```python
from build123d import *

# Parameters (mm, degrees)
ANGLE_BRACKET_DEPTH = 24.765
CORNERS_R           = 5.08
SKETCH2_R           = 2.2225
HOLES_DEPTH         = 32.661678194
SLOTS_DEPTH         = 32.710646251


with BuildPart() as part:
    # Sketch1 → Angle Bracket (new body)
    with BuildSketch(Plane.XY):
        with BuildLine():
            Line((0, 13.589), (0, 1.27))
            ThreePointArc((0, 1.27), (0.371974388, 0.371974388), (1.27, 0))
            Line((1.27, 0), (15.24, 0))
            Line((15.24, 0), (15.24, 0.9398))
            Line((15.24, 0.9398), (1.8796, 0.9398))
            ThreePointArc((1.8796, 0.9398), (1.215061047, 1.215061047), (0.9398, 1.8796))
            Line((0.9398, 1.8796), (0.9398, 13.589))
            Line((0.9398, 13.589), (0, 13.589))
        make_face()
    extrude(amount=-ANGLE_BRACKET_DEPTH)

    # Corners
    corners_edges = [part.edges().sort_by_distance(p)[0] for p in [
        (0.4699, 13.589, 0),
        (15.24, 0.4699, -24.765),
        (0.4699, 13.589, -24.765),
        (15.24, 0.4699, 0),
    ]]
    fillet(corners_edges, radius=CORNERS_R)

    # Sketch2 → Holes (cut, through all)
    with BuildSketch(Plane(origin=(0.9398, 0, 0), x_dir=(0, 0, -1), z_dir=(1, 0, 0))):
        with Locations(Location((6.0325, 7.5565, 0), (0, 0, 90))):
            Circle(SKETCH2_R)
        with Locations(Location((18.7325, 7.5565, 0), (0, 0, 90))):
            Circle(SKETCH2_R)
    extrude(amount=-HOLES_DEPTH, mode=Mode.SUBTRACT)

    # Sketch3 → Slots (cut, through all)
    with BuildSketch(Plane(origin=(0, 0.9398, 0), x_dir=(-1, 0, 0), z_dir=(0, 1, 0))):
        with BuildLine():
            Line((-5.3975, -3.81), (-9.2075, -3.81))
            ThreePointArc((-9.2075, -3.81), (-11.43, -6.0325), (-9.2075, -8.255))
            Line((-9.2075, -8.255), (-5.3975, -8.255))
            ThreePointArc((-5.3975, -8.255), (-3.175, -6.0325), (-5.3975, -3.81))
        make_face()
        with BuildLine():
            Line((-5.3975, -16.51), (-9.2075, -16.51))
            ThreePointArc((-9.2075, -16.51), (-11.43, -18.7325), (-9.2075, -20.955))
            Line((-9.2075, -20.955), (-5.3975, -20.955))
            ThreePointArc((-5.3975, -20.955), (-3.175, -18.7325), (-5.3975, -16.51))
        make_face()
    extrude(amount=-SLOTS_DEPTH, mode=Mode.SUBTRACT)


solid = part.part
```
Source: CAD feature listing. Evaluate the final solid. Frame: model axes, mm. A direction names the side the tool comes from. Round coordinates to 2 decimals unless told otherwise and drop trailing zeros. Order: outer loops, then holes, each group sorted by start corner. A loop starts at its lowest first (then second) coordinate and runs counter-clockwise, first axis right, second up. Notation, with made-up numbers: (68, 17) -> (114, 17) arc R33 cw to (114, 52) -> close; hole circle Ø1 at (38, 34.5). An arc over 180 degrees is marked (long way). One line per item, written item: value. Start each with the question number.
Q1. Access query for faces 4 (the flat face through (2.8, 0.5, 0)), 5 (the flat face through (7.3, 0.5, -3.81)). Directions: +Z, -Z, +X, -X, +Y, -Y. A direction counts if a zero-diameter tool reaches every point of the face in a straight line with its end or side. Return the directions, or none.
Q2. Section query A-A (x = 6.5). Return the cut outline in (y, z) (3 decimals), plus the area to 3 significant figures.
Q3. Section query C-C (y = 9). Return the cut outline in (x, z).
Q4. Section query D-D (z = -11.5). Return the cut outline in (x, y).
Q5. Material intervals for probe 1 along X at (y, z) = (4.5, -19.75); probe 2 along Y at (x, z) = (1.5, -8.25), sorted ascending.
Q6. Pin query (flat end, axial travel): pin 1 (3 mm diameter, centred on y = 5, z = -10.5, fed in from +X); pin 2 (4 mm diameter, centred on y = 7.56, z = -6.03, fed in from +X); pin 3 (1 mm diameter, centred on x = 7.5, z = -8.5, fed in from +Y). Return the tip coordinate at first contact, or that it passes through.
Q7. Draft query along X for faces 1 (the flat face through (7.3, 0.5, -20.955)), 2 (the flat face through (0.94, 8, -12)), 3 (the flat face through (9, 0.94, -12)). Return one class per face: pulls with the +X half, pulls with the -X half, needs draft (parallel to the pull), parting line crosses it, or undercut.
Q8. Section query B-B (z = -17.5). Return the cut outline in (x, y), plus the area to 3 significant figures.
Findings below:
1. face 4: +Z, +X, -X, +Y, -Y
1. face 5: +Y, -Y
2. outline: (0, -24.765) -> (0.94, -24.765) -> (0.94, -20.955) -> (0, -20.955) -> close; (0, -16.51) -> (0.94, -16.51) -> (0.94, -8.255) -> (0, -8.255) -> close; (0, -3.81) -> (0.94, -3.81) -> (0.94, 0) -> (0, 0) -> close
2. area: 14.9 mm²
3. outline: (0, -24.74) -> (0.94, -24.74) -> (0.94, -20.42) -> (0, -20.42) -> close; (0, -17.04) -> (0.94, -17.04) -> (0.94, -7.72) -> (0, -7.72) -> close; (0, -4.34) -> (0.94, -4.34) -> (0.94, -0.02) -> (0, -0.02) -> close
4. outline: (0, 1.27) arc R1.27 ccw to (1.27, 0) -> (15.24, 0) -> (15.24, 0.94) -> (1.88, 0.94) arc R0.94 cw to (0.94, 1.88) -> (0.94, 13.59) -> (0, 13.59) -> close
5. probe 1: 0 to 0.94
5. probe 2: 0 to 1.02
6. pin 1: x = 0.94
6. pin 2: through
6. pin 3: y = 0.94
7. face 1: undercut
7. face 2: pulls with the +X half
7. face 3: needs draft
8. outline: (0, 1.27) arc R1.27 ccw to (1.27, 0) -> (3.55, 0) -> (3.55, 0.94) -> (1.88, 0.94) arc R0.94 cw to (0.94, 1.88) -> (0.94, 5.71) -> (0, 5.71) -> close; (0, 9.41) -> (0.94, 9.41) -> (0.94, 13.59) -> (0, 13.59) -> close; (11.06, 0) -> (15.24, 0) -> (15.24, 0.94) -> (11.06, 0.94) -> close
8. area: 15.5 mm²
